Check sheet for the modelled part. Datum: model origin and axes. Units: mm. Face numbers are marked on the shaded views. A direction names the side the tool comes from. Give positions to 0.01 mm unless a question says otherwise; leave off trailing zeros. Loops run counter-clockwise (first coordinate to the right, second up) from the corner with the lowest first, then second, coordinate; pieces in that order, holes last. Notation, with made-up numbers: M 23,11.5 L 75,11.5 A24 cw 75,46.5 Z; hole C 51,72 d4. An arc over 180 degrees is marked long. Write each question's results on one line, items separated by ' | '. Start each with the question number.
1. Sectioned sample at B-B on z = 8. Record the cut outline in (x, y).
2. Sectioned sample at D-D on x = 48. Record the cut outline in (y, z).
3. Tool access check on the marked faces 4, 5 and 6. Record the directions out of +Z, -Z, +X, -X, +Y, -Y that give a thin tool (end or side, any length) a straight path to the whole face; none if there is none.
4. Draft check along X on the marked faces 1, 2 and 3. Enter one of: pulls with the +X half, pulls with the -X half, needs draft (parallel to the pull), parting line crosses it, or undercut.
5. Go/stop test with a flat-tipped pin: pin 1 (1.8 mm diameter, centred on y = 3.5, z = 5, fed in from +X). Record where the tip stops, or that it passes through.
6. Sectioned sample at A-A on z = 18.5. Record the cut outline in (x, y), and give its area (3 significant figures).
7. Material ranges on line 1 along Z through (x, y) = (23.5, 3.45); line 2 along X through (y, z) = (4.25, 8.5); line 3 along X through (y, z) = (3.45, -17.5), recorded low to high.
8. Sectioned sample at C-C on x = -2.5. Record the cut outline in (y, z).
```python
from build123d import *

# Parameters (mm, degrees)
SKETCH1_W           = 62
SKETCH1_H           = 54
SKETCH1_W_2         = 27
SKETCH1_H_2         = 14
BOSS_EXTRUDE1_DEPTH = 6
SKETCH2_R           = 0.75
CUT_EXTRUDE1_DEPTH  = 63.417946137
SKETCH3_R           = 1.75
CUT_EXTRUDE2_DEPTH  = 63.417946137
FILLET1_R           = 3
SKETCH4_W           = 16
SKETCH4_H           = 12
CUT_EXTRUDE3_DEPTH  = 63.417946137


with BuildPart() as part:
    # Sketch1 → Boss-Extrude1 (new body)
    with BuildSketch(Plane(origin=(0, 0, 0), x_dir=(1, 0, 0), z_dir=(0, 1, 0))):
        with Locations((21, -7)):
            Rectangle(SKETCH1_W, SKETCH1_H)
        with Locations((13.5, -7)):
            Rectangle(SKETCH1_W_2, SKETCH1_H_2, mode=Mode.SUBTRACT)
    extrude(amount=BOSS_EXTRUDE1_DEPTH)

    # Sketch2 → Cut-Extrude1 (cut, through all)
    with BuildSketch(Plane(origin=(0, 6, 0), x_dir=(1, 0, 0), z_dir=(0, 1, 0))):
        with Locations(Location((-2.5, 3.75, 0), (0, 0, 270))):
            Circle(SKETCH2_R)
        with Locations(Location((-2.5, -18.5, 0), (0, 0, 270))):
            Circle(SKETCH2_R)
        with Locations(Location((26.5, 3, 0), (0, 0, 270))):
            Circle(SKETCH2_R)
        with Locations(Location((26.5, -18.5, 0), (0, 0, 270))):
            Circle(SKETCH2_R)
    extrude(amount=-CUT_EXTRUDE1_DEPTH, mode=Mode.SUBTRACT)

    # Sketch3 → Cut-Extrude2 (cut, through all)
    with BuildSketch(Plane(origin=(0, 6, 0), x_dir=(1, 0, 0), z_dir=(0, 1, 0))):
        with Locations(Location((-6, 16, 0), (0, 0, 270))):
            Circle(SKETCH3_R)
        with Locations(Location((-6, -30, 0), (0, 0, 270))):
            Circle(SKETCH3_R)
        with Locations(Location((48, 16, 0), (0, 0, 270))):
            Circle(SKETCH3_R)
        with Locations(Location((48, -30, 0), (0, 0, 270))):
            Circle(SKETCH3_R)
    extrude(amount=-CUT_EXTRUDE2_DEPTH, mode=Mode.SUBTRACT)

    # Fillet1
    fillet1_edges = [part.edges().sort_by_distance(p)[0] for p in [
        (-10, 3, -20),
        (52, 3, -20),
        (52, 3, 34),
        (-10, 3, 34),
    ]]
    fillet(fillet1_edges, radius=FILLET1_R)

    # Sketch4 → Cut-Extrude3 (cut, through all)
    with BuildSketch(Plane(origin=(0, 6, 0), x_dir=(1, 0, 0), z_dir=(0, 1, 0))):
        with Locations((52, -7)):
            Rectangle(SKETCH4_W, SKETCH4_H)
    extrude(amount=-CUT_EXTRUDE3_DEPTH, mode=Mode.SUBTRACT)


solid = part.part
```
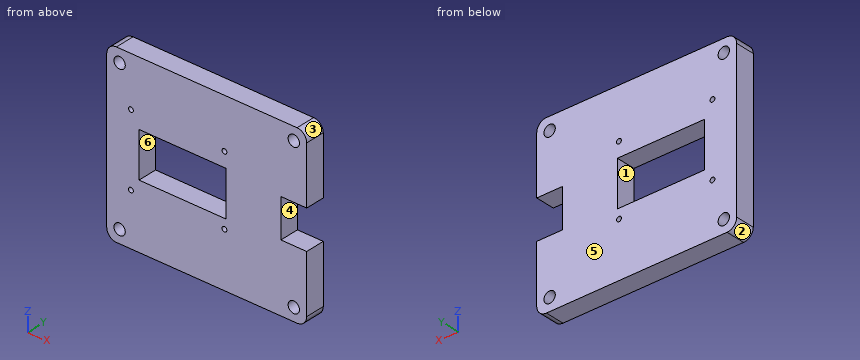
Output values:
1) outline: M -10,0 L 0,0 L 0,6 L -10,6 Z; M 27,0 L 44,0 L 44,6 L 27,6 Z
2) outline: M 0,-20 L 6,-20 L 6,-17.75 L 0,-17.75 Z; M 0,-14.25 L 6,-14.25 L 6,1 L 0,1 Z; M 0,13 L 6,13 L 6,28.25 L 0,28.25 Z; M 0,31.75 L 6,31.75 L 6,34 L 0,34 Z
3) face 4: +X, +Y, -Y | face 5: +Z, -Z, +X, -X, +Y | face 6: +Y, -Y
4) face 1: undercut | face 2: pulls with the -X half | face 3: pulls with the +X half
5) pin 1: x = 44
6) outline: M -10,0 L -3.25,0 L -3.25,6 L -10,6 Z; M -1.75,0 L 25.75,0 L 25.75,6 L -1.75,6 Z; M 27.25,0 L 52,0 L 52,6 L 27.25,6 Z | area: 354 mm2
7) line 1: -20 to 0, 14 to 34 | line 2: -10 to 0, 27 to 44 | line 3: -9.96 to -6.9, -5.1 to 47.1, 48.9 to 51.96
8) outline: M 0,-20 L 6,-20 L 6,-4.5 L 0,-4.5 Z; M 0,-3 L 6,-3 L 6,17.75 L 0,17.75 Z; M 0,19.25 L 6,19.25 L 6,34 L 0,34 Z
